CAD build for the part. Positions are in the model's coordinates, mm. Face numbers are marked on the shaded views. A direction names the side the tool comes from. Coordinates: 2 decimals unless noted, no trailing zeros. Write each loop counter-clockwise with the first axis right and the second up, starting at its lowest first coordinate (ties: lowest second). Pieces come first, ordered by that corner, then holes. Notation, with made-up numbers: (14.5, -7.75) -> (54.5, -7.75) arc R16 ccw to (54.5, 13.25) -> close; hole circle Ø2 at (47.5, -21). An arc over 180 degrees is marked (long way). Answer as CSV lines item,"result". Start each with the question number.
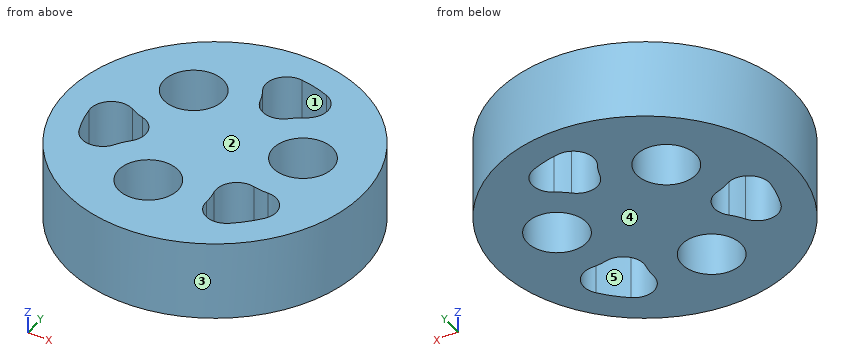
Autodesk Inventor part; units mm, degrees
ref_plane "YZ Plane" through (0, 0, 0) normal (1, 0, 0) x (0, 1, 0)
ref_plane "XZ Plane" through (0, 0, 0) normal (0, 1, 0) x (-1, 0, 0)
ref_plane "XY Plane" through (0, 0, 0) normal (0, 0, 1) x (1, 0, 0)
sketch "スケッチ1" plane through (0, 0, 0) normal (0, 0, 1) x (1, 0, 0)
  circle A0 centre (0, 0) radius 6.975
  circle A1 centre (-2.8284, 2.8284) radius 1.5
  circle A2 centre (-1.0353, -3.8637) radius 1.5
  circle A3 centre (3.8637, 1.0353) radius 1.5
  circle A4 centre (0, 0) radius 7.5
  dimension "d0" = 13.95
  dimension "d1" = 3
  dimension "d2" = 4
  dimension "d5" = 360
  dimension "d9" = 15
extrude "押し出し2" add sketch "スケッチ1" along normal blind 4 contours A0 | A4
sketch "スケッチ2" plane through (0, 0, 4) normal (0, 0, 1) x (1, 0, 0)
  circle A0 centre (0, 0) radius 7.5
  circle A1 centre (-1.0353, -3.8637) radius 1.5
  circle A2 centre (-2.8284, 2.8284) radius 1.5
  circle A3 centre (3.8637, 1.0353) radius 1.5
  circle A4 centre (0, 0) radius 3
  circle A5 centre (0, 0) radius 6
  circle A6 centre (-2.8284, 2.8284) radius 3
  circle A7 centre (-1.0353, -3.8637) radius 3
  circle A8 centre (3.8637, 1.0353) radius 3
  point P0 (5.882, -1.1843)
  point P1 (2.5106, -1.6422)
  point P2 (1.6422, -2.5106)
  point P3 (1.1843, -5.882)
  point P4 (1.3531, 2.6775)
  point P5 (4.5018, 3.9666)
  point P6 (-1.9153, 5.6861)
  point P7 (0.1669, 2.9954)
  point P8 (-3.9666, -4.5018)
  point P9 (-2.6775, -1.3531)
  point P10 (-2.9954, -0.1669)
  point P11 (-5.6861, 1.9153)
  dimension "d13" = 6
  dimension "d14" = 1.5
  dimension "d15" = 1.5
  dimension "d16" = 1.5
  dimension "d17" = 1.5
extrude "押し出し3" cut sketch "スケッチ2" against normal blind 10 contours A4 A8 A5 A7 | A7 A5 A6 A4 | A4 A6 A5 A8
fillet "フィレット1" radius 1.05 12 edges at (-1.9153, 5.6861, 2) (4.5018, 3.9666, 2) (0.1669, 2.9954, 2) (1.3531, 2.6775, 2) (-5.6861, 1.9153, 2) (-2.9954, -0.1669, 2) (-2.6775, -1.3531, 2) (-3.9666, -4.5018, 2) (2.5106, -1.6422, 2) (1.6422, -2.5106, 2) (5.882, -1.1843, 2) (1.1843, -5.882, 2)
properties part number "アームカムD15t4" material "アセタール樹脂、白"
1. Cut at A-A (y = 0.75). Give the cut face in (x, z).
2. Flat gauge pins, fed straight in: P1, Ø2, axis at x = -2, z = 0.5, coming from the -Y side; P2, Ø1.5, axis at y = 2.5, z = 0.5, coming from the -X side. Where does each tip first touch, or does it go through?
3. Cut at C-C (x = -6.25). Give the cut face in (y, z), then the cut area to 3 significant figures.
4. Tool access for the marked faces 4 and 5: list every direction of +Z, -Z, +X, -X, +Y, -Y with a clear straight run to the whole face (end or side of a thin tool).
5. Mould opens along Y. For the marked faces 1, 2 and 3 say: pulls with the +Y half, pulls with the -Y half, needs draft (parallel to the pull), parting line crosses it, or undercut.
6. Cut at B-B (y = 4). Count the separate pieces of the cut face and the enclosed holes in it, then the cut area to 3 significant figures.
7. Wall check: line 1 (Y direction, x = -1.5, z = 1.3); line 2 (X direction, y = -3.5, z = 1.15); line 3 (X direction, y = -0.25, z = 0.5). Give the ranges that are in metal, low to high.
Geometry check:
1,outline,"(-7.46, 0) -> (2.39, 0) -> (2.39, 4) -> (-7.46, 4) -> close; (5.34, 0) -> (7.46, 0) -> (7.46, 4) -> (5.34, 4) -> close"
2,P1,"y = -7.43"
2,P2,"x = -7.29"
3,outline,"(-4.15, 0) -> (4.15, 0) -> (4.15, 4) -> (-4.15, 4) -> close"
3,area,"33.2 mm²"
4,face 4,"-Z, +X, -X, +Y, -Y"
4,face 5,"+Z, -Z"
5,face 1,"undercut"
5,face 2,"needs draft"
5,face 3,"parting line crosses it"
6,separate pieces,"3"
6,enclosed holes,"0"
6,area,"31.9 mm²"
7,line 1,"-7.35 to -5.29, -2.44 to 2.13, 3.53 to 7.35"
7,line 2,"-6.63 to -2.49, 0.42 to 1.94, 4.86 to 6.63"
7,line 3,"-7.5 to -5.88, -3.29 to 3.09, 4.64 to 7.5"
